Part model, mm, in its own coordinate system. Coordinates: 2 decimals unless noted, no trailing zeros. Loops run counter-clockwise (first coordinate to the right, second up) from the corner with the lowest first, then second, coordinate; pieces in that order, holes last. Notation, with made-up numbers: M -39,-38.75 L -2,-38.75 A12 cw -2,-25.75 Z; hole C 14.5,-19 d10. An arc over 180 degrees is marked long. Answer as a JSON object with one key per item and string values. Group by question number.
1. Saw through at D-D on z = -49. Write the cut outline in (x, y), then the cut area to 3 significant figures.
2. Drill centre lines: L1, parallel to X at y = 1.7, z = 8; L2, parallel to Z at x = 25, y = 0.2; L3, parallel to Z at x = -20, y = 1.7. Where is each one in solid material? Low to high.
3. Drop flat-ended pins along their axis: pin 1 Ø1 at (x, y) = (35.5, 1.5) entering from +Z; pin 2 Ø1.2 at (y, z) = (2.5, 3) entering from +X; pin 3 Ø4 at (x, z) = (-22, 8) entering from +Y; pin 4 Ø1.5 at (y, z) = (0.5, -38.5) entering from -X. Give the stop position or say it passes through.
4. Saw through at B-B on x = 16. Write the cut outline in (y, z), then the cut area to 3 significant figures.
5. Saw through at A-A on z = 8. Write the cut outline in (x, y).
6. Saw through at C-C on y = 2.4. Count the separate pieces of the cut face and the enclosed holes in it, then the cut area to 3 significant figures.
from build123d import *

# Parameters (mm, degrees)
EXTRUDE_1_DEPTH     = 4
FILLET_1_R          = 10
FILLET_2_R          = 5
SKETCH_2_R          = 2.6
CUT_EXTRUDE_1_DEPTH = 62.032778079
SKETCH_3_R          = 1.6
CUT_EXTRUDE_2_DEPTH = 62.032778079
EXTRUDE_2_DEPTH     = 4
FILLET_3_R          = 2


with BuildPart() as part:
    # 草图1 → 凸台-拉伸1 (new body)
    with BuildSketch(Plane(origin=(0, 0, 0), x_dir=(1, 0, 0), z_dir=(0, 1, 0))):
        Polygon((-30, -15), (30, -15), (30, 15), (20, 35), (20, 43), (24, 47), (24, 53), (12, 53), (-5, 19.408174518), (-30, 15), align=None)
    extrude(amount=EXTRUDE_1_DEPTH)

    # 圆角1
    fillet_1_edges = [part.edges().sort_by_distance(p)[0] for p in [
        (-5, 2, -19.408174518),
    ]]
    fillet(fillet_1_edges, radius=FILLET_1_R)

    # 圆角2
    fillet_2_edges = [part.edges().sort_by_distance(p)[0] for p in [
        (30, 2, -15),
        (30, 2, 15),
        (-30, 2, 15),
        (-30, 2, -15),
        (12, 2, -53),
        (20, 2, -35),
    ]]
    fillet(fillet_2_edges, radius=FILLET_2_R)

    # 草图2 → 切除-拉伸1 (cut, through all)
    with BuildSketch(Plane(origin=(0, 4, 0), x_dir=(1, 0, 0), z_dir=(0, 1, 0))):
        with Locations(Location((-22, 8, 0), (0, 0, 270))):
            Circle(SKETCH_2_R)
        with Locations(Location((22, 8, 0), (0, 0, 90))):
            Circle(SKETCH_2_R)
        with Locations(Location((22, -8, 0), (0, 0, 270))):
            Circle(SKETCH_2_R)
        with Locations(Location((-22, -8, 0), (0, 0, 90))):
            Circle(SKETCH_2_R)
    extrude(amount=-CUT_EXTRUDE_1_DEPTH, mode=Mode.SUBTRACT)

    # 草图3 → 切除-拉伸2 (cut, through all)
    with BuildSketch(Plane.XZ):
        with Locations(Location((16, -49, 0), (0, 0, 270))):
            Circle(SKETCH_3_R)
    extrude(amount=-CUT_EXTRUDE_2_DEPTH, mode=Mode.SUBTRACT)

    # 草图4 → 凸台-拉伸2 (add)
    with BuildSketch(Plane(origin=(0, 4, 0), x_dir=(1, 0, 0), z_dir=(0, 1, 0))):
        Polygon((24, 47), (32, 47), (32, 31), (38, 31), (38, 53), (24, 53), align=None)
    extrude(amount=-EXTRUDE_2_DEPTH)

    # 圆角3
    fillet_3_edges = [part.edges().sort_by_distance(p)[0] for p in [
        (38, 2, -53),
        (38, 2, -31),
        (32, 2, -31),
        (32, 2, -47),
        (24, 2, -47),
        (20, 2, -43),
    ]]
    fillet(fillet_3_edges, radius=FILLET_3_R)


solid = part.part
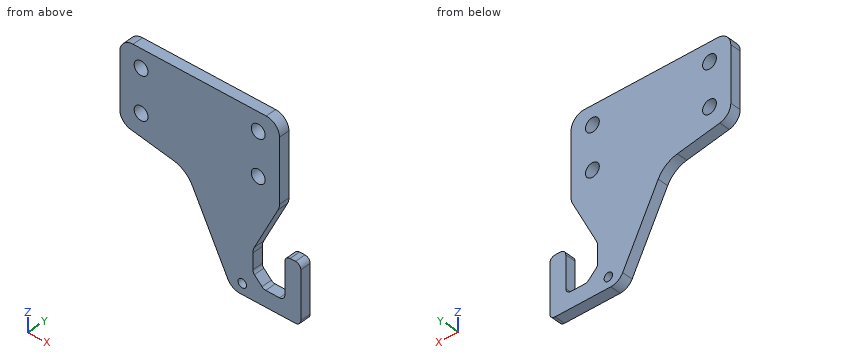
Outcome:
{
 "1": {"outline": "M 9.98,0 L 14.4,0 L 14.4,4 L 9.98,4 Z; M 17.6,0 L 38,0 L 38,4 L 17.6,4 Z", "area": "99.3 mm²"},
 "2": {"L1": "x = -30 to -24.6, -19.4 to 19.4, 24.6 to 30", "L2": "z = -53 to -47, -25 to 15", "L3": "z = -16.76 to -9.66, -6.34 to 6.34, 9.66 to 15"},
 "3": {"pin 1": "stops at z = -31", "pin 2": "stops at x = 30", "pin 3": "passes through", "pin 4": "stops at x = 4.28"},
 "4": {"outline": "M 0,-53 L 4,-53 L 4,-50.6 L 0,-50.6 Z; M 0,-47.4 L 4,-47.4 L 4,15 L 0,15 Z", "area": "259 mm²"},
 "5": {"outline": "M -30,0 L -24.6,0 L -24.6,4 L -30,4 Z; M -19.4,0 L 19.4,0 L 19.4,4 L -19.4,4 Z; M 24.6,0 L 30,0 L 30,4 L 24.6,4 Z"},
 "6": {"separate pieces": "1", "enclosed holes": "5", "area": "2,720 mm²"}
}
